```python
from build123d import *

# Parameters (mm, degrees)
SKETCH1_R                                           = 30
SKETCH1_R_2                                         = 6.5
BOSS_EXTRUDE1_DEPTH                                 = 5
CSK_FOR_M3_COUNTERSUNK_FLAT_HEAD_SCREW1_D           = 3.4
CSK_FOR_M3_COUNTERSUNK_FLAT_HEAD_SCREW1_DEPTH       = 5
CSK_FOR_M3_COUNTERSUNK_FLAT_HEAD_SCREW1_CSINK_D     = 6.3
CSK_FOR_M3_COUNTERSUNK_FLAT_HEAD_SCREW1_CSINK_ANGLE = 90
CSK_FOR_M3_COUNTERSUNK_FLAT_HEAD_SCREW2_D           = 3.4
CSK_FOR_M3_COUNTERSUNK_FLAT_HEAD_SCREW2_DEPTH       = 5
CSK_FOR_M3_COUNTERSUNK_FLAT_HEAD_SCREW2_CSINK_D     = 6.3
CSK_FOR_M3_COUNTERSUNK_FLAT_HEAD_SCREW2_CSINK_ANGLE = 90


with BuildPart() as part:
    # Sketch1 → Boss-Extrude1 (new body)
    with BuildSketch(Plane(origin=(0, 0, 0), x_dir=(1, 0, 0), z_dir=(0, 1, 0))):
        Circle(SKETCH1_R)
        Circle(SKETCH1_R_2, mode=Mode.SUBTRACT)
    extrude(amount=BOSS_EXTRUDE1_DEPTH)

    # CSK for M3 Countersunk Flat Head Screw1
    with Locations(Plane(origin=(0, 5, 0), x_dir=(1, 0, 0), z_dir=(0, 1, 0))):
        with Locations((0, 25), (-25, 0), (0, -25), (25, 0)):
            CounterSinkHole(CSK_FOR_M3_COUNTERSUNK_FLAT_HEAD_SCREW1_D / 2, CSK_FOR_M3_COUNTERSUNK_FLAT_HEAD_SCREW1_CSINK_D / 2, depth=CSK_FOR_M3_COUNTERSUNK_FLAT_HEAD_SCREW1_DEPTH, counter_sink_angle=CSK_FOR_M3_COUNTERSUNK_FLAT_HEAD_SCREW1_CSINK_ANGLE)

    # CSK for M3 Countersunk Flat Head Screw2
    with Locations(Plane(origin=(0, 0, 0), x_dir=(-1, 0, 0), z_dir=(0, -1, 0))):
        with Locations((0, 11.5), (-11.5, 0), (0, -11.5), (11.5, 0)):
            CounterSinkHole(CSK_FOR_M3_COUNTERSUNK_FLAT_HEAD_SCREW2_D / 2, CSK_FOR_M3_COUNTERSUNK_FLAT_HEAD_SCREW2_CSINK_D / 2, depth=CSK_FOR_M3_COUNTERSUNK_FLAT_HEAD_SCREW2_DEPTH, counter_sink_angle=CSK_FOR_M3_COUNTERSUNK_FLAT_HEAD_SCREW2_CSINK_ANGLE)


solid = part.part
```
Check sheet for the modelled part. Datum: model origin and axes. Units: mm. Round coordinates to 2 decimals unless told otherwise and drop trailing zeros. Order: outer loops, then holes, each group sorted by start corner. A loop starts at its lowest first (then second) coordinate and runs counter-clockwise, first axis right, second up. Notation, with made-up numbers: M 31,9 L 88,9 A25 ccw 88,33 Z; hole C 86.25,44 d5. An arc over 180 degrees is marked long. Answer in a Markdown table with one row per item.
(1) Section check A-A on x = 0. Give the number of separate pieces and of enclosed holes in the cut face, plus the area to 3 significant figures.
Findings:
| item | result |
|---|---|
| separate pieces | 6 |
| enclosed holes | 0 |
| area | 159 mm^2 |
(2) Section check D-D on x = -25. Record the boundary of the cut face in (y, z).
Findings:
| item | result |
|---|---|
| outline | M 0,-16.58 L 5,-16.58 L 5,-3.15 L 3.55,-1.7 L 0,-1.7 Z; M 0,1.7 L 3.55,1.7 L 5,3.15 L 5,16.58 L 0,16.58 Z |
(3) Section check C-C on z = -11.5. Record the boundary of the cut face in (x, y).
Findings:
| item | result |
|---|---|
| outline | M -27.71,0 L -3.15,0 L -1.7,1.45 L -1.7,5 L -27.71,5 Z; M 1.7,1.45 L 3.15,0 L 27.71,0 L 27.71,5 L 1.7,5 Z |
(4) Material ranges on line 1 along X through (y, z) = (2.3, 0); line 2 along X through (y, z) = (3.05, 11.5), recorded low to high. Write a range as from..to.
Findings:
| item | result |
|---|---|
| line 1 | x = -30..-26.7, -23.3..-13.2, -9.8..-6.5, 6.5..9.8, 13.2..23.3, 26.7..30 |
| line 2 | x = -27.71..-1.7, 1.7..27.71 |
(5) Gauge pin test, flat ends, axial feed: pin 1 (1.5 mm diameter, centred on x = 19, y = 3, fed in from -Z); pin 2 (5.5 mm diameter, centred on x = 0, z = -25, fed in from +Y); pin 3 (1 mm diameter, centred on y = 2, z = 1, fed in from -X); pin 4 (1.5 mm diameter, centred on x = -21.5, z = 0.5, fed in from -Y). Record the tip position at first contact, or that the pin passes through.
Findings:
| item | result |
|---|---|
| pin 1 | stops at z = -23.81 |
| pin 2 | stops at y = 4.6 |
| pin 3 | stops at x = -30 |
| pin 4 | stops at y = 0 |
(6) Draft check along Z on faces 1 (the cylindrical face through (-0.221, 3.25, -13.186)), 2 (the cylindrical face through (-29.97, 2.46, -1.32)), 3 (the flat face through (0, 0, -7)). Enter one of: +Z half, -Z half, draft (parallel to the pull), parting line (faces both ways), or undercut.
Findings:
| item | result |
|---|---|
| face 1 | undercut |
| face 2 | parting line |
| face 3 | draft |
